Geometry: final body of the model. Coordinates: model frame, mm. Face numbers are marked on the shaded views. A direction names the side the tool comes from. Coordinates: 2 decimals unless noted, no trailing zeros. Write each loop counter-clockwise with the first axis right and the second up, starting at its lowest first coordinate (ties: lowest second). Pieces come first, ordered by that corner, then holes. Notation, with made-up numbers: M 67,-29 L 108,-29 A26 ccw 108,-11 Z; hole C 4.5,45.25 d1. An arc over 180 degrees is marked long. Write item = value, one per line. Start each with the question number.
Item 1: Section B-B on z = 21. Output: boundary loops of the cut face in (x, y).
Item 2: Reachability of the marked faces 1 and 2 from +Z, -Z, +X, -X, +Y, -Y: full face, straight path, thin tool, end or side. Return the list, or none.
Item 3: Section C-C on x = 11. Output: boundary loops of the cut face in (y, z).
Item 4: Section A-A on y = -66. Output: boundary loops of the cut face in (x, z).
Item 5: First-contact query: pin 1 Ø3.5 at (y, z) = (-62, 5) entering from +X; pin 2 Ø5.5 at (x, y) = (17.5, -75.5) entering from +Z; pin 3 Ø1 at (y, z) = (-133, 19.5) entering from +X; pin 4 Ø12 at (x, y) = (6, -86.5) entering from +Z. Flat tips, straight axial feed; report the tip coordinate or a pass-through.
Item 6: Ray query, L1, parallel to X at y = -35.5, z = 23.25; L2, parallel to Z at x = 4.5, y = -148.5; L3, parallel to X at y = -152, z = 5. Return the intervals inside material, ascending. Write a range as [from, to].
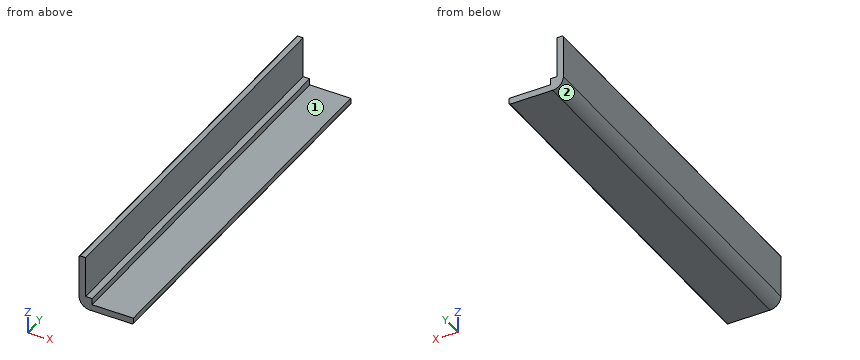
from build123d import *

# Parameters (mm, degrees)
F1_DEPTH = 176.666666
F2_R     = 5
F3_R     = 0.5


with BuildPart() as f1:
    # F0 (on Front) → F1 (new body)
    with BuildSketch(Plane.XZ):
        Polygon((3, 25), (0, 25), (0, 0), (25, 0), (25, 3), (6, 3), (6, 6), (3, 6), align=None)
    extrude(amount=F1_DEPTH)

    # F2
    f2_edges = [f1.edges().sort_by_distance(p)[0] for p in [
        (0, -88.333333, 0),
    ]]
    fillet(f2_edges, radius=F2_R)

    # F3
    f3_edges = [f1.edges().sort_by_distance(p)[0] for p in [
        (0, -88.333333, 25),
        (25, -88.333333, 0),
    ]]
    fillet(f3_edges, radius=F3_R)


solid = f1.part
Responses:
q1.outline = M 0,-176.67 L 3,-176.67 L 3,0 L 0,0 Z
q2.face_1 = +Z, +X, +Y, -Y
q2.face_2 = -Z, -X, +Y, -Y
q3.outline = M -176.67,0 L 0,0 L 0,3 L -176.67,3 Z
q4.outline = M 0,5 A5 ccw 5,0 L 24.5,0 A0.5 ccw 25,0.5 L 25,3 L 6,3 L 6,6 L 3,6 L 3,25 L 0.5,25 A0.5 ccw 0,24.5 Z
q5.pin_1 = 6
q5.pin_2 = 3
q5.pin_3 = 3
q5.pin_4 = 25
q6.L1 = [0, 3]
q6.L2 = [0.03, 6]
q6.L3 = [0, 6]
